Geometry check sheet. Reference: the model listing, model coordinates, mm. Face numbers are marked on the shaded views. A direction names the side the tool comes from. Coordinates: 2 decimals unless noted, no trailing zeros. Write each loop counter-clockwise with the first axis right and the second up, starting at its lowest first coordinate (ties: lowest second). Pieces come first, ordered by that corner, then holes.
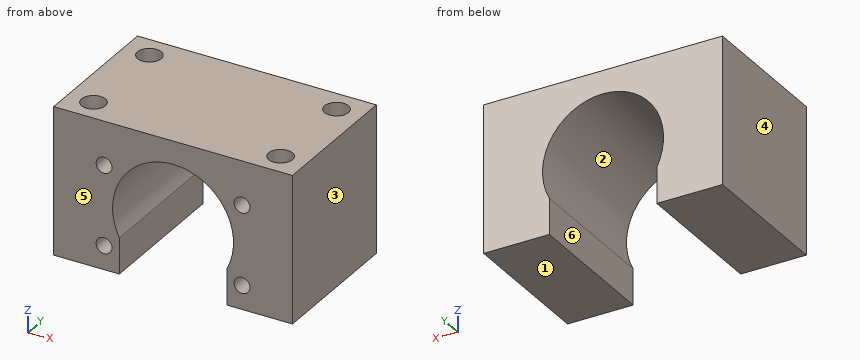
from build123d import *

# Parameters (mm, degrees)
F1_DEPTH = 18
F2_R     = 2
F4_DEPTH = 10
F3_R     = 3
F5_DEPTH = 16


with BuildPart() as f1:
    # F0 (on Front) → F1 (new body, symmetric)
    with BuildSketch(Plane.XZ):
        with BuildLine():
            ThreePointArc((-13.5, -6.984984), (0, 15.2), (13.5, -6.984984))
            Line((13.5, -6.984984), (13.5, -16))
            Line((13.5, -16), (30, -16))
            Line((30, -16), (30, 21))
            Line((30, 21), (-30, 21))
            Line((-30, 21), (-30, -16))
            Line((-30, -16), (-13.5, -16))
            Line((-13.5, -16), (-13.5, -6.984984))
        make_face()
    extrude(amount=F1_DEPTH, both=True)

    # F2 (on face) → F4 (cut)
    with BuildSketch(Plane.XZ.offset(18)):
        with Locations((-17.320508, 10)):
            Circle(F2_R)
        with Locations((17.320508, 10)):
            Circle(F2_R)
        with Locations((17.320508, -10)):
            Circle(F2_R)
        with Locations((-17.320508, -10)):
            Circle(F2_R)
    extrude(amount=-F4_DEPTH, mode=Mode.SUBTRACT)

    # F3 (on face) → F5 (cut)
    with BuildSketch(Plane.XY.offset(21)):
        with Locations((-23.5, 12)):
            Circle(F3_R)
        with Locations((23.5, 12)):
            Circle(F3_R)
        with Locations((23.5, -12)):
            Circle(F3_R)
        with Locations((-23.5, -12)):
            Circle(F3_R)
    extrude(amount=-F5_DEPTH, mode=Mode.SUBTRACT)


solid = f1.part
1. Sectioned sample at B-B, the plane y = -12. Record the boundary of the cut face in (x, z).
Computed values:
outline: (-30, -16) - (-13.5, -16) - (-13.5, -6.98) arc R15.2 cw (long way) to (13.5, -6.98) - (13.5, -16) - (30, -16) - (30, 21) - (26.5, 21) - (26.5, 5) - (20.5, 5) - (20.5, 21) - (-20.5, 21) - (-20.5, 5) - (-26.5, 5) - (-26.5, 21) - (-30, 21) - close; hole circle Ø4 at (-17.32, -10); hole circle Ø4 at (-17.32, 10); hole circle Ø4 at (17.32, -10); hole circle Ø4 at (17.32, 10)
2. Sectioned sample at A-A, the plane z = 10. Record the boundary of the cut face in (x, y), and give its area (3 significant figures).
Computed values:
outline: (-30, -18) - (-19.32, -18) - (-19.32, -8) - (-15.32, -8) - (-15.32, -18) - (-11.45, -18) - (-11.45, 18) - (-30, 18) - close; (11.45, -18) - (15.32, -18) - (15.32, -8) - (19.32, -8) - (19.32, -18) - (30, -18) - (30, 18) - (11.45, 18) - close; hole circle Ø6 at (-23.5, -12); hole circle Ø6 at (-23.5, 12); hole circle Ø6 at (23.5, -12); hole circle Ø6 at (23.5, 12)
area: 1,140 mm2
3. Sectioned sample at C-C, the plane x = -23.5. Record the boundary of the cut face in (y, z).
Computed values:
outline: (-18, -16) - (18, -16) - (18, 21) - (15, 21) - (15, 5) - (9, 5) - (9, 21) - (-9, 21) - (-9, 5) - (-15, 5) - (-15, 21) - (-18, 21) - close
4. Thickness scan on line 1 along Y through (x, z) = (23.5, 15.5); line 2 along X through (y, z) = (9, 0); line 3 along X through (y, z) = (-9.5, -13). Record the ranges inside material, lowest first.
Computed values:
line 1: y = -18 to -15, -9 to 9, 15 to 18
line 2: x = -30 to -15.2, 15.2 to 30
line 3: x = -30 to -13.5, 13.5 to 30
5. Gauge pin test, flat ends, axial feed: pin 1 Ø3 at (x, y) = (-22.5, 11) entering from +Z; pin 2 Ø3 at (x, z) = (-17, -10.5) entering from -Y; pin 3 Ø1.2 at (x, z) = (17.5, -10.5) entering from -Y. Record the tip position at first contact, or that the pin passes through.
Computed values:
pin 1: stops at z = 5
pin 2: stops at y = -18
pin 3: stops at y = -8
6. Draft check along X on the marked faces 1, 2, 3 and 4. Enter one of: released by +X, released by -X, zero draft, split by the parting line, or undercut.
Computed values:
face 1: zero draft
face 2: undercut
face 3: released by +X
face 4: released by -X
7. Access from +Z, -Z, +X, -X, +Y, -Y to the whole of each face (thin tool, end or side, straight path). Record for the marked faces 5 and 6.
Computed values:
face 5: +Z, -Z, +X, -X, -Y
face 6: -Z, +Y, -Y
8. Sectioned sample at D-D, the plane y = 12. Record the boundary of the cut face in (x, z).
Computed values:
outline: (-30, -16) - (-13.5, -16) - (-13.5, -6.98) arc R15.2 cw (long way) to (13.5, -6.98) - (13.5, -16) - (30, -16) - (30, 21) - (26.5, 21) - (26.5, 5) - (20.5, 5) - (20.5, 21) - (-20.5, 21) - (-20.5, 5) - (-26.5, 5) - (-26.5, 21) - (-30, 21) - close
